Could you check a few things on this model? Use its own coordinates, in mm. Round coordinates to 2 decimals unless told otherwise and drop trailing zeros. Write each loop counter-clockwise with the first axis right and the second up, starting at its lowest first coordinate (ties: lowest second). Pieces come first, ordered by that corner, then holes. Notation, with made-up numbers: (-35.5, 3) - (-15.5, 3) arc R18 ccw to (-15.5, 11) - close; hole circle Ø10 at (30.5, 45.25). An arc over 180 degrees is marked (long way). Put each result on its own line as item: value.
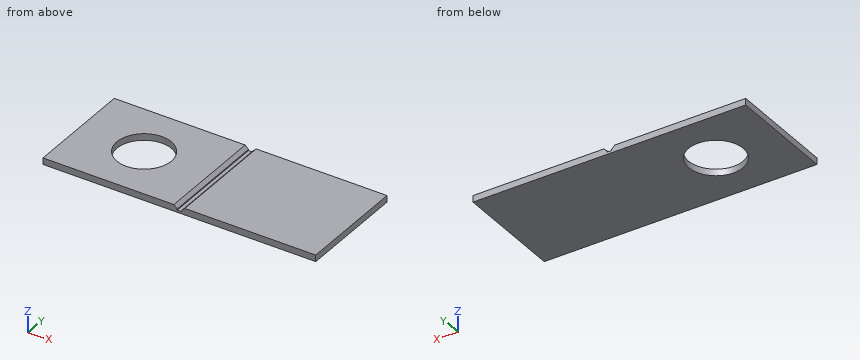
from build123d import *

# Parameters (mm, degrees)
F0_W     = 50
F0_H     = 20
F1_DEPTH = 0.4
F2_W     = 24.6
F2_H     = 20
F3_DEPTH = 0.8
F4_R     = 5
F5_DEPTH = 25
F6_SIZE  = 0.6


with BuildPart() as f1:
    # F0 (on Top) → F1 (new body)
    with BuildSketch(Plane.XY):
        Rectangle(F0_W, F0_H)
    extrude(amount=F1_DEPTH)

    # F2 (on face) → F3 (join)
    with BuildSketch(Plane.XY.offset(0.4)):
        with Locations((-12.7, 0)):
            Rectangle(F2_W, F2_H)
        with Locations((12.7, 0)):
            Rectangle(F2_W, F2_H)
    extrude(amount=F3_DEPTH)

    # F4 (on face) → F5 (cut)
    with BuildSketch(Plane.XY.offset(1.2)):
        with Locations((-13, 0)):
            Circle(F4_R)
    extrude(amount=-F5_DEPTH, mode=Mode.SUBTRACT)

    # F6
    f6_edges = [f1.edges().sort_by_distance(p)[0] for p in [
        (-0.4, 0, 1.2),
        (0.4, 0, 1.2),
    ]]
    chamfer(f6_edges, length=F6_SIZE)


solid = f1.part
(1) Please list where these lines run through material, in increasing order: probe 1 along X at (y, z) = (-0.25, 0.45); probe 2 along Y at (x, z) = (-13, 0.6); probe 3 along X at (y, z) = (-1.5, 0.75). Write a range as from..to.
Values found:
probe 1: x = -25..-17.99, -8.01..-0.4, 0.4..25
probe 2: y = -10..-5, 5..10
probe 3: x = -25..-17.77, -8.23..-0.55, 0.55..25
(2) Imagine slicing it at C-C, the plane y = 0. List the corners of the cut face in (x, z) for me.
Values found:
outline: (-25, 0) - (-18, 0) - (-18, 1.2) - (-25, 1.2) - close; (-8, 0) - (25, 0) - (25, 1.2) - (1, 1.2) - (0.4, 0.6) - (0.4, 0.4) - (-0.4, 0.4) - (-0.4, 0.6) - (-1, 1.2) - (-8, 1.2) - close
(3) Imagine slicing it at D-D, the plane y = -5.75. List the corners of the cut face in (x, z) for me, then the cut area to 3 significant figures.
Values found:
outline: (-25, 0) - (25, 0) - (25, 1.2) - (1, 1.2) - (0.4, 0.6) - (0.4, 0.4) - (-0.4, 0.4) - (-0.4, 0.6) - (-1, 1.2) - (-25, 1.2) - close
area: 59.0 mm^2
(4) I'm going to push flat-ended pins straight in: pin 1 (12 mm diameter, centred on x = 13.5, y = 6.5, fed in from -Z); pin 2 (0.6 mm diameter, centred on x = 0, y = 3.5, fed in from +Z). Where does each tip first touch, or does it pass through?
Values found:
pin 1: stops at z = 0
pin 2: stops at z = 0.4
(5) Imagine slicing it at A-A, the plane z = 0.8. List the corners of the cut face in (x, y) for me.
Values found:
outline: (-25, -10) - (-0.6, -10) - (-0.6, 10) - (-25, 10) - close; (0.6, -10) - (25, -10) - (25, 10) - (0.6, 10) - close; hole circle Ø10 at (-13, 0)
(6) Imagine slicing it at B-B, the plane x = -13. List the corners of the cut face in (y, z) for me, then the cut area to 3 significant figures.
Values found:
outline: (-10, 0) - (-5, 0) - (-5, 1.2) - (-10, 1.2) - close; (5, 0) - (10, 0) - (10, 1.2) - (5, 1.2) - close
area: 12.0 mm^2
